Geometry check sheet. Reference: the model listing, model coordinates, mm. A direction names the side the tool comes from. Coordinates: 2 decimals unless noted, no trailing zeros. Loops run counter-clockwise (first coordinate to the right, second up) from the corner with the lowest first, then second, coordinate; pieces in that order, holes last. Notation, with made-up numbers: M 13.5,30.25 L 70.5,30.25 A18 cw 70.5,36.25 Z; hole C 83,64.5 d4. An arc over 180 degrees is marked long. Use CSV: the item, a comma, the result in double quotes.
Solid Edge part; units mm, degrees
sketch "Sketch1" plane through (0, 0, 0) normal (0, 0, 1) x (1, 0, 0)
  circle A0 centre (0, 0) radius 6
extrude "Protrusion1" add sketch "Sketch1" along normal mid plane 100
chamfer "Chamfer1" distance 0.9 angle 45 2 edges at (-6, 0, -50) (-6, 0, 50)
sketch "Sketch2" plane through (0, 0, 50) normal (0, 0, 1) x (1, 0, 0)
  line L0 (-1.7321, 3) -> (1.7321, 3)
  line L1 (3.4641, 0) -> (1.7321, 3)
  line L2 (1.7321, -3) -> (3.4641, 0)
  line L3 (-1.7321, -3) -> (1.7321, -3)
  line L4 (-3.4641, 0) -> (-1.7321, -3)
  line L5 (-1.7321, 3) -> (-3.4641, 0)
extrude "Cutout1" cut sketch "Sketch2" against normal blind 50
properties part number "123532"
1. Section check C-C, the plane z = -38. Record the cut outline in (x, y).
The answers:
outline,"C 0,0 d12"
2. Gauge pin test, flat ends, axial feed: P1, Ø2, axis at y = -3.5, z = -7.5, coming from the -X side; P2, Ø1.8, axis at x = 1, y = 1, coming from the +Z side; P3, Ø4, axis at x = 4.5, z = 36, coming from the -Y side. Record the tip position at first contact, or that the pin passes through.
The answers:
P1,"x = -5.45"
P2,"z = 0"
P3,"y = -5.45"
3. Release check for a two-part mould opening along X. For faces 1 (the cylindrical face through (-6, 0, -1)), 2 (the flat face through (2.6, -1.5, 25.4)), 3 (the flat face through (-0.1, -3.3, 50)) record: +X half, -X half, draft (parallel to the pull), parting line (faces both ways), or undercut.
The answers:
face 1,"parting line"
face 2,"undercut"
face 3,"draft"
4. Section check B-B, the plane x = 0. Record the cut outline in (y, z).
The answers:
outline,"M -6,-49.1 L -5.1,-50 L 5.1,-50 L 6,-49.1 L 6,49.1 L 5.1,50 L 3,50 L 3,0 L -3,0 L -3,50 L -5.1,50 L -6,49.1 Z"
5. Set-up check for faces 4 (the flat face through (0, 0, 0)), 5 (the flat face through (0, 0, -50)): record each of +Z, -Z, +X, -X, +Y, -Y from which the full face is reachable in a straight line by a thin tool's end or side.
The answers:
face 4,"+Z"
face 5,"-Z, +X, -X, +Y, -Y"
6. Thickness scan on line 1 (Y direction, x = 0.25, z = 17); line 2 (Z direction, x = 2.5, y = -1.25); line 3 (X direction, y = -2, z = 23.5). Record the ranges inside material, lowest first. Write a range as [from, to].
The answers:
line 1,"[-5.99, -3], [3, 5.99]"
line 2,"[-50, 0]"
line 3,"[-5.66, -2.31], [2.31, 5.66]"
7. Section check A-A, the plane z = 3.5. Record the cut outline in (x, y), plus the area to 3 significant figures.
The answers:
outline,"C 0,0 d12; hole M -3.46,0 L -1.73,-3 L 1.73,-3 L 3.46,0 L 1.73,3 L -1.73,3 Z"
area,"81.9 mm^2"
